Source: three-view drawing plus pictorial views. Frame: mm from the lowest corner of the part. Coordinates: 2 decimals unless noted, no trailing zeros. Write each loop counter-clockwise with the first axis right and the second up, starting at its lowest first coordinate (ties: lowest second). Pieces come first, ordered by that corner, then holes. Notation, with made-up numbers: (72.25, 75.25) - (95.25, 75.25) arc R15 ccw to (95.25, 96.25) - close; hole circle Ø5 at (69.25, 10). An arc over 180 degrees is marked (long way). Put each result on its own line as item: value.
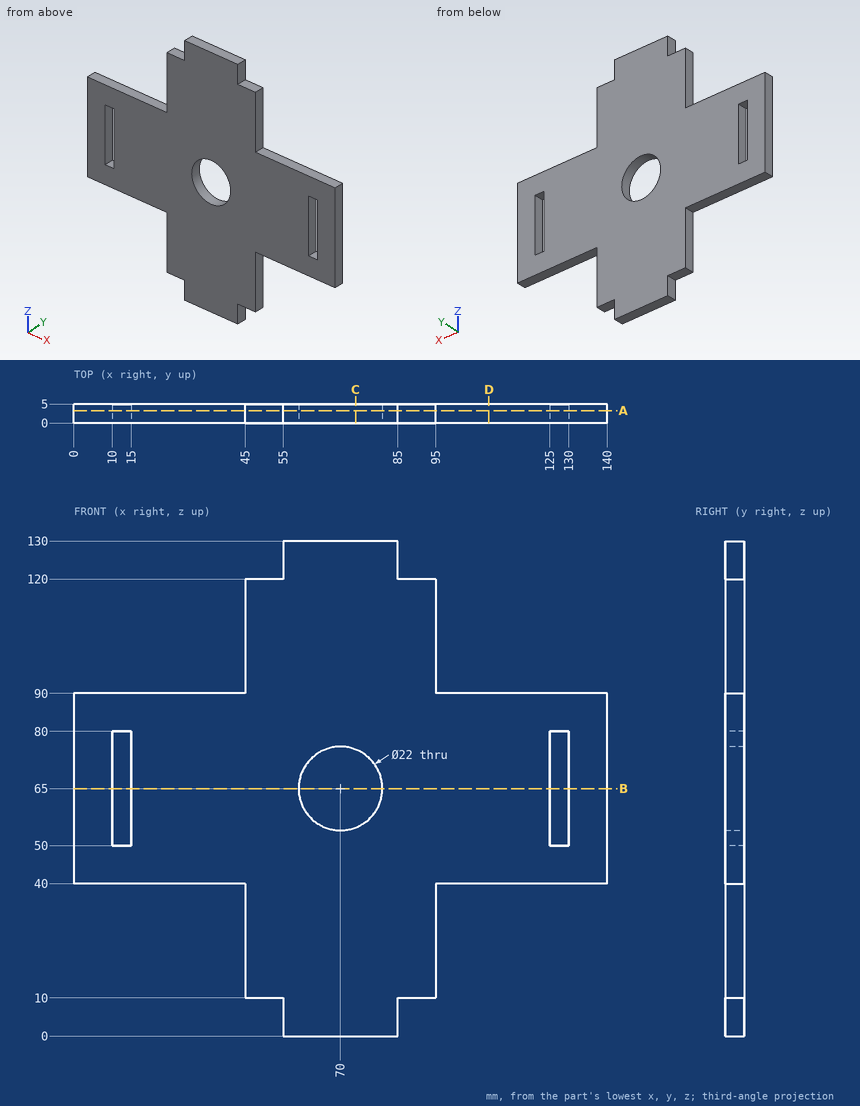
1. Pin query (flat end, axial travel): pin 1 Ø1.5 at (y, z) = (2.5, 104.5) entering from -X; pin 2 Ø1.5 at (x, y) = (126.5, 1.5) entering from +Z; pin 3 Ø1.5 at (x, y) = (125, 1.5) entering from -Z. Return the tip coordinate at first contact, or that it passes through.
Answer below:
pin 1: stops at x = 45
pin 2: stops at z = 90
pin 3: stops at z = 40
2. Ray query, probe 1 along X at (y, z) = (2.6, 65); probe 2 along X at (y, z) = (4.45, 51.5); probe 3 along X at (y, z) = (0.5, 71). Return the intervals inside material, ascending. Write a range as from..to.
Answer below:
probe 1: x = 0..10, 15..59, 81..125, 130..140
probe 2: x = 0..10, 15..125, 130..140
probe 3: x = 0..10, 15..60.78, 79.22..125, 130..140
3. Section query D-D (x = 109). Return loops of the section in (y, z), then the cut area to 3 significant figures.
Answer below:
outline: (0, 40) - (5, 40) - (5, 90) - (0, 90) - close
area: 250 mm²
4. Section query C-C (x = 74). Return loops of the section in (y, z), then the cut area to 3 significant figures.
Answer below:
outline: (0, 0) - (5, 0) - (5, 54.75) - (0, 54.75) - close; (0, 75.25) - (5, 75.25) - (5, 130) - (0, 130) - close
area: 548 mm²
5. Section query A-A (y = 3.25). Count the separate pieces of the cut face and the enclosed holes in it, then the cut area to 3 significant figures.
Answer below:
separate pieces: 1
enclosed holes: 3
area: 9,920 mm²
6. Section query B-B (z = 65). Return loops of the section in (x, y), then the cut area to 3 significant figures.
Answer below:
outline: (0, 0) - (10, 0) - (10, 5) - (0, 5) - close; (15, 0) - (59, 0) - (59, 5) - (15, 5) - close; (81, 0) - (125, 0) - (125, 5) - (81, 5) - close; (130, 0) - (140, 0) - (140, 5) - (130, 5) - close
area: 540 mm²
